Geometry check sheet. Reference: the model listing, model coordinates, mm. A direction names the side the tool comes from. Round coordinates to 2 decimals unless told otherwise and drop trailing zeros. Loops run counter-clockwise (first coordinate to the right, second up) from the corner with the lowest first, then second, coordinate; pieces in that order, holes last. Notation, with made-up numbers: (46.25, -17) -> (87.25, -17) arc R9 ccw to (87.25, -5) -> close; hole circle Ø2 at (58.25, 55.5). An arc over 180 degrees is marked (long way). Use one line per item in the form item = value.
from build123d import *

# Parameters (mm, degrees)
F1_DEPTH = 63.5
F2_DEPTH = 9.525
F3_DEPTH = 38.1
F5_R     = 6.35


with BuildPart() as f1:
    # F0 (on Front) → F1 (new body, symmetric)
    with BuildSketch(Plane.XZ):
        Polygon((47.625, 19.05), (-66.675, 19.05), (-66.675, -19.05), (66.675, -19.05), (66.675, 19.05), align=None)
    extrude(amount=F1_DEPTH, both=True)

    # F0 (on Front) → F2 (join, symmetric)
    with BuildSketch(Plane.XZ):
        with BuildLine():
            add(Edge.make_bspline(
                [(-66.675, 19.05), (-45.088604, 71.2366), (17.616627, 83.509553), (78.066317, 92.984823)],
                knots=[0, 0, 0, 0, 163.406627, 163.406627, 163.406627, 163.406627], degree=3))
            Line((-66.675, 19.05), (47.625, 19.05))
            Line((47.625, 19.05), (47.625, 50.8))
            ThreePointArc((47.625, 50.8), (56.029969, 76.810734), (78.066317, 92.984823))
        make_face()
    extrude(amount=F2_DEPTH, both=True)

    # F0 (on Front) → F3 (join, symmetric)
    with BuildSketch(Plane.XZ):
        with BuildLine():
            Line((47.625, 50.8), (47.625, 19.05))
            Line((47.625, 19.05), (66.675, 19.05))
            Line((66.675, 19.05), (66.675, 50.8))
            ThreePointArc((66.675, 50.8), (74.269175, 68.913879), (92.510638, 76.196264))
            Line((92.510638, 76.196264), (120.014986, 76.196264))
            Line((120.014986, 76.196264), (120.014986, 95.246264))
            Line((120.014986, 95.246264), (92.651304, 95.246264))
            add(Edge.make_bspline(
                [(78.066317, 92.984823), (82.950328, 93.750374), (87.819616, 94.497663), (92.651304, 95.246264)],
                knots=[163.406627, 163.406627, 163.406627, 163.406627, 176.609009, 176.609009, 176.609009, 176.609009], degree=3))
            ThreePointArc((78.066317, 92.984823), (56.029969, 76.810734), (47.625, 50.8))
        make_face()
    extrude(amount=F3_DEPTH, both=True)

    # F0 (on Front) → F4 (revolve)
    with BuildSketch(Plane.XZ):
        Polygon((120.014986, 102.023325), (120.014986, 95.246264), (136.960638, 95.246264), (136.960638, 76.196264), (120.014986, 76.196264), (120.014986, 63.923325), (158.114986, 63.923325), (158.114986, 102.023325), align=None)
    revolve(axis=Axis((120.014986, 0, 82.973325), (0, 0, -1)))

    # F5
    f5_edges = [f1.edges().sort_by_distance(p)[0] for p in [
        (-66.675, -63.5, 0),
        (66.675, -63.5, 0),
        (66.675, 63.5, 0),
        (-66.675, 63.5, 0),
    ]]
    fillet(f5_edges, radius=F5_R)


solid = f1.part
1. Gauge pin test, flat ends, axial feed: pin 1 (22 mm diameter, centred on x = 12.5, z = 38.5, fed in from +Y) (3 decimals); pin 2 (12 mm diameter, centred on y = -45.5, z = 25, fed in from +X) (3 decimals); pin 3 (5.5 mm diameter, centred on y = -7.5, z = 81.5, fed in from +X). Record the tip position at first contact, or that the pin passes through.
Return value:
pin_1 = 9.525
pin_2 = 66.675
pin_3 = 157.82
2. Mould release check, pull along Y, two halves, no side actions. Record for faces 6 (the cylindrical face through (155.21, 14.59, 83.24)), 7 (the flat face through (127, 0, 95.246)), 8 (the flat face through (99, -34, 95.246)), 9 (the flat face through (126, 0, 76.196)): released by +Y, released by -Y, zero draft, split by the parting line, or undercut.
Return value:
face_6 = split by the parting line
face_7 = undercut
face_8 = zero draft
face_9 = undercut
3. Section check B-B (x = 139.5). Record the boundary of the cut face in (y, z), then the cut area to 3 significant figures.
Return value:
outline = (-32.74, 63.92) -> (32.74, 63.92) -> (32.74, 102.02) -> (-32.74, 102.02) -> close
area = 2,490 mm2
4. Section check A-A (z = -9). Record the boundary of the cut face in (x, y) (3 decimals), then the cut area to 3 significant figures.
Return value:
outline = (-66.675, -57.15) arc R6.35 ccw to (-60.325, -63.5) -> (60.325, -63.5) arc R6.35 ccw to (66.675, -57.15) -> (66.675, 57.15) arc R6.35 ccw to (60.325, 63.5) -> (-60.325, 63.5) arc R6.35 ccw to (-66.675, 57.15) -> close
area = 16,900 mm2
5. Tool access check on faces 1 (the flat face through (-1, 63.5, 0)), 2 (the cylindrical face through (64.864, -61.59, 0.267)), 3 (the flat face through (47.625, -24, 35)), 4 (the flat face through (99, 34, 95.246)), 5 (the flat face through (121, -1, 63.923)). Record the directions out of +Z, -Z, +X, -X, +Y, -Y that give a thin tool (end or side, any length) a straight path to the whole face; none if there is none.
Return value:
face_1 = +Z, -Z, +X, -X, +Y
face_2 = +Z, -Z, +X, -Y
face_3 = +Z, -X, -Y
face_4 = +Z, -X, +Y
face_5 = -Z, +X, +Y, -Y
6. Material ranges on line 1 along Z through (x, y) = (117, 1); line 2 along X through (y, z) = (-35, 31.5) (3 decimals); line 3 along Z through (x, y) = (62.5, -51.5), recorded low to high.
Return value:
line_1 = 63.92 to 102.02
line_2 = 47.625 to 66.675
line_3 = -19.05 to 19.05
